from build123d import *

# Parameters (mm, degrees)
SKETCH1_W           = 14.8
SKETCH1_H           = 4.8
SKETCH1_R           = 1.6
BOSS_EXTRUDE1_DEPTH = 4
CUT_EXTRUDE2_DEPTH  = 0.4
SKETCH3_R           = 1.6
SKETCH3_R_2         = 1.1
BOSS_EXTRUDE2_DEPTH = 1
FILLET1_R           = 0.4


with BuildPart() as part:
    # Sketch1 → Boss-Extrude1 (new body)
    with BuildSketch(Plane(origin=(0, 0, 0), x_dir=(1, 0, 0), z_dir=(0, 1, 0))):
        Rectangle(SKETCH1_W, SKETCH1_H)
        with Locations(Location((-5, 0, 0), (0, 0, 270))):
            Circle(SKETCH1_R, mode=Mode.SUBTRACT)
        with Locations(Location((5, 0, 0), (0, 0, 270))):
            Circle(SKETCH1_R, mode=Mode.SUBTRACT)
    extrude(amount=BOSS_EXTRUDE1_DEPTH)

    # Sketch2 → Cut-Extrude2 (cut)
    with BuildSketch(Plane.XZ):
        with BuildLine():
            Line((-5, -2.4), (5, -2.4))
            ThreePointArc((5, -2.4), (2.6, 0), (5, 2.4))
            Line((5, 2.4), (-5, 2.4))
            ThreePointArc((-5, 2.4), (-2.6, 0), (-5, -2.4))
        make_face()
    extrude(amount=-CUT_EXTRUDE2_DEPTH, mode=Mode.SUBTRACT)

    # Sketch3 → Boss-Extrude2 (add)
    # profile 1 of 2: a face of its own
    with BuildSketch(Plane.XZ):
        with Locations(Location((5, 0, 0), (0, 0, 90))):
            Circle(SKETCH3_R)
        with Locations(Location((5, 0, 0), (0, 0, 270))):
            Circle(SKETCH3_R_2, mode=Mode.SUBTRACT)
    # profile 2 of 2: a face of its own
    with BuildSketch(Plane.XZ):
        with Locations(Location((-5, 0, 0), (0, 0, 90))):
            Circle(SKETCH3_R)
        with Locations(Location((-5, 0, 0), (0, 0, 270))):
            Circle(SKETCH3_R_2, mode=Mode.SUBTRACT)
    extrude(amount=-BOSS_EXTRUDE2_DEPTH)

    # Fillet1
    fillet1_edges = [part.edges().sort_by_distance(p)[0] for p in [
        (-7.4, 2, -2.4),
        (7.4, 2, -2.4),
        (7.4, 2, 2.4),
        (-7.4, 2, 2.4),
    ]]
    fillet(fillet1_edges, radius=FILLET1_R)


solid = part.part
Work out the finished part from the listing and answer in its coordinate system (mm). A direction names the side the tool comes from. Give positions to 0.01 mm unless a question says otherwise; leave off trailing zeros. Loops run counter-clockwise (first coordinate to the right, second up) from the corner with the lowest first, then second, coordinate; pieces in that order, holes last. Notation, with made-up numbers: (10, 60.25) -> (15, 60.25) arc R6 cw to (15, 64.25) -> close; hole circle Ø2 at (43, -10). An arc over 180 degrees is marked (long way). Use a Markdown table: item, result. Add a question column.
1. Section A-A on y = 2.2 is taken. Determine the outline of the cut face in (x, z).
2. For faces 4 (the flat face through (7.4, 2, 0)), 5 (the cylindrical face through (-6.56, 2.48, -0.35)), 6 (the cylindrical face through (2.6, 0.2, -0.05)), determine the directions among +Z, -Z, +X, -X, +Y, -Y from which every point of the face is accessible in a straight line to the end or side of a thin tool.
3. Section B-B on z = 0 is taken. Determine the outline of the cut face in (x, y).
4. Section C-C on x = 5.5 is taken. Determine the outline of the cut face in (y, z).
5. Determine the mould class of faces 1 (the flat face through (-7.4, 2, 0)), 2 (the cylindrical face through (3.44, 2.48, -0.35)), 3 (the flat face through (-6, 0, -1)) for opening direction X: released by +X, released by -X, zero draft, split by the parting line, or undercut.
6. Section D-D on z = 1.3 is taken. Determine the outline of the cut face in (x, y).
7. Find the intervals of material crossed by probe 1 along X at (y, z) = (0.8, 0); probe 2 along Z at (x, y) = (5, 3.4); probe 3 along X at (y, z) = (1.5, -0.45), in increasing order.
Results below:
| question | item | result |
|---|---|---|
| 1 | outline | (-7.4, -2) arc R0.4 ccw to (-7, -2.4) -> (7, -2.4) arc R0.4 ccw to (7.4, -2) -> (7.4, 2) arc R0.4 ccw to (7, 2.4) -> (-7, 2.4) arc R0.4 ccw to (-7.4, 2) -> close; hole circle Ø3.2 at (-5, 0); hole circle Ø3.2 at (5, 0) |
| 2 | face 4 | +Z, -Z, +X, +Y, -Y |
| 2 | face 5 | +Y |
| 2 | face 6 | -Y |
| 3 | outline | (-7.4, 0) -> (-6.1, 0) -> (-6.1, 1) -> (-6.6, 1) -> (-6.6, 4) -> (-7.4, 4) -> close; (-3.9, 0) -> (-2.6, 0) -> (-2.6, 0.4) -> (2.6, 0.4) -> (2.6, 0) -> (3.9, 0) -> (3.9, 1) -> (3.4, 1) -> (3.4, 4) -> (-3.4, 4) -> (-3.4, 1) -> (-3.9, 1) -> close; (6.1, 0) -> (7.4, 0) -> (7.4, 4) -> (6.6, 4) -> (6.6, 1) -> (6.1, 1) -> close |
| 4 | outline | (0, -2.4) -> (4, -2.4) -> (4, -1.52) -> (1, -1.52) -> (1, -0.98) -> (0, -0.98) -> close; (0, 0.98) -> (1, 0.98) -> (1, 1.52) -> (4, 1.52) -> (4, 2.4) -> (0, 2.4) -> close |
| 5 | face 1 | released by -X |
| 5 | face 2 | undercut |
| 5 | face 3 | zero draft |
| 6 | outline | (-7.4, 0) -> (-2.98, 0) -> (-2.98, 0.4) -> (2.98, 0.4) -> (2.98, 0) -> (7.4, 0) -> (7.4, 4) -> (5.93, 4) -> (5.93, 1) -> (4.07, 1) -> (4.07, 4) -> (-4.07, 4) -> (-4.07, 1) -> (-5.93, 1) -> (-5.93, 4) -> (-7.4, 4) -> close |
| 7 | probe 1 | x = -7.4 to -6.1, -3.9 to 3.9, 6.1 to 7.4 |
| 7 | probe 2 | z = -2.4 to -1.6, 1.6 to 2.4 |
| 7 | probe 3 | x = -7.4 to -6.54, -3.46 to 3.46, 6.54 to 7.4 |
